```python
from build123d import *

# Parameters (mm, degrees)
BOSS_EXTRUDE1_DEPTH = 60
CUT_EXTRUDE2_DEPTH  = 1
CUT_EXTRUDE3_DEPTH  = 40
CUT_EXTRUDE4_DEPTH  = 10
SKETCH9_R           = 3
CUT_EXTRUDE5_DEPTH  = 1


with BuildPart() as part:
    # Sketch1 → Boss-Extrude1 (new body)
    with BuildSketch(Plane.XY):
        Polygon((-15, 1), (15, 1), (0, -24.980762114), align=None)
        Polygon((-13.267949192, 0), (13.267949192, 0), (0, -22.980762114), align=None, mode=Mode.SUBTRACT)
    extrude(amount=BOSS_EXTRUDE1_DEPTH)

    # Sketch4 → Cut-Extrude2 (cut)
    with BuildSketch(Plane(origin=(10.816987298, -6.245190528, 0), x_dir=(0, 0, -1), z_dir=(0.8660254037844365, -0.500000000000004, 0))):
        with BuildLine():
            Line((-60, 8.366025404), (-60, -21.633974596))
            add(Edge.make_bspline(
                [(-60, -21.633974596), (-29.886538221, -24.240664674), (-20, 8.366025404)],
                knots=[0, 0, 0, 1, 1, 1], degree=2))
            Line((-20, 8.366025404), (-60, 8.366025404))
        make_face()
    cut_extrude2 = extrude(amount=-CUT_EXTRUDE2_DEPTH, mode=Mode.SUBTRACT)

    # Mirror1: Cut-Extrude2 across plane
    add(cut_extrude2.mirror(Plane(origin=(0, 0, 0), x_dir=(0, 0, 1), z_dir=(1, 0, 0))), mode=Mode.SUBTRACT)

    # Sketch5 → Cut-Extrude3 (cut)
    with BuildSketch(Plane.XY.offset(60)):
        Polygon((-13.845299459, 0.999999995), (13.845299462, 1), (13.267949197, 8e-09), (-13.267949192, 0), align=None)
    extrude(amount=-CUT_EXTRUDE3_DEPTH, mode=Mode.SUBTRACT)

    # Sketch8 → Cut-Extrude4 (cut)
    with BuildSketch(Plane(origin=(0, 0, 0), x_dir=(-1, 0, 0), z_dir=(0, 0, -1))):
        Polygon((-15.872166784, 0), (15.872166784, 0), (0, -24.980762114), align=None)
    extrude(amount=-CUT_EXTRUDE4_DEPTH, mode=Mode.SUBTRACT)

    # Sketch9 → Cut-Extrude5 (cut)
    with BuildSketch(Plane(origin=(0, 1, 0), x_dir=(1, 0, 0), z_dir=(0, 1, 0))):
        with Locations((0, -2)):
            Circle(SKETCH9_R)
    extrude(amount=-CUT_EXTRUDE5_DEPTH, mode=Mode.SUBTRACT)


solid = part.part
```
CAD build for the part. Positions are in the model's coordinates, mm. A direction names the side the tool comes from. Give positions to 0.01 mm unless a question says otherwise; leave off trailing zeros. Loops run counter-clockwise (first coordinate to the right, second up) from the corner with the lowest first, then second, coordinate; pieces in that order, holes last. Notation, with made-up numbers: (6, 35) - (17, 35) arc R17 ccw to (17, 64) - close; hole circle Ø8 at (-17, 25.25). An arc over 180 degrees is marked (long way). Put each result on its own line as item: value.
Q1. Tool access for faces 1 (the face through (0.2, 0.5, 20)), 2 (the face through (-5.4, -14.3, 10)), 3 (the face through (0, 1, 10)): list every direction of +Z, -Z, +X, -X, +Y, -Y with a clear straight run to the whole face (end or side of a thin tool).
Filled in:
face 1: +Z, +Y
face 2: -Z, +X, -X, -Y
face 3: +Z, -Z, +X, -X, +Y
Q2. Probe line 1 along Y through (x, z) = (-12, 12); line 2 along X through (y, z) = (0.7, 2); line 3 along X through (y, z) = (0.2, 2). List the from-to ranges inside material, lowest first.
Filled in:
line 1: y = -4.2 to -2.2, 0 to 1
line 2: x = -14.83 to -3, 3 to 14.83
line 3: x = -14.54 to -3, 3 to 14.54
Q3. Flat gauge pins, fed straight in: pin 1 (1.5 mm diameter, centred on x = 6, y = -14.5, fed in from -Z); pin 2 (5 mm diameter, centred on x = 0, z = 2, fed in from -Y); pin 3 (3 mm diameter, centred on x = -2.5, z = 40.5, fed in from +Y); pin 4 (1.1 mm diameter, centred on x = 3, y = 0.5, fed in from +Z). Where does each tip first touch, or does it go through?
Filled in:
pin 1: stops at z = 10
pin 2: passes through
pin 3: stops at y = -21.89
pin 4: stops at z = 20
Q4. Slice it at A-A (z = 2). Give the cut face in (x, y), plus the area to 3 significant figures.
Filled in:
outline: (-15, 1) - (-14.42, 0) - (-3, 0) - (-3, 1) - close; (3, 0) - (14.42, 0) - (15, 1) - (3, 1) - close
area: 23.4 mm²
Q5. Slice it at B-B (z = 8). Give the cut face in (x, y), plus the area to 3 significant figures.
Filled in:
outline: (-15, 1) - (-14.42, 0) - (14.42, 0) - (15, 1) - close
area: 29.4 mm²
Q6. Mould opens along X. For faces 4 (the face through (-8.5, 0.5, 0)), 5 (the face through (-5.798, -14.938, 21.826)), 6 (the face through (0, 0, 10)) say: pulls with the +X half, pulls with the -X half, needs draft (parallel to the pull), parting line crosses it, or undercut.
Filled in:
face 4: needs draft
face 5: pulls with the -X half
face 6: undercut
